```python
from build123d import *

# Parameters (mm, degrees)
SKETCH1_W                                    = 240
SKETCH1_H                                    = 100
BOSS_EXTRUDE1_DEPTH                          = 5
SKETCH2_W                                    = 20
SKETCH2_H                                    = 5
BOSS_EXTRUDE2_DEPTH                          = 5
MIRROR1_AT_THE_SECOND_PLANE_COPY_1_SKETC_W   = 20
MIRROR1_AT_THE_SECOND_PLANE_COPY_1_SKETC_H   = 5
MIRROR1_AT_THE_SECOND_PLANE_COPY_1_DEPTH     = 5
SKETCH3_R                                    = 6
SKETCH3_R_2                                  = 2
BOSS_EXTRUDE3_DEPTH                          = 5
SKETCH4_R                                    = 2.5
CUT_EXTRUDE2_DEPTH                           = 5
MIRROR2_AT_THE_SECOND_PLANE_COPY_1_SKETC_R   = 6
MIRROR2_AT_THE_SECOND_PLANE_COPY_1_SKETC_R_2 = 2
MIRROR2_AT_THE_SECOND_PLANE_COPY_1_DEPTH     = 5
MIRROR2_AT_THE_SECOND_PLANE_COPY_2_SKETC_R   = 2.5
MIRROR2_AT_THE_SECOND_PLANE_COPY_2_DEPTH     = 5


with BuildPart() as part:
    # Sketch1 → Boss-Extrude1 (new body)
    with BuildSketch(Plane.XY):
        Rectangle(SKETCH1_W, SKETCH1_H)
    extrude(amount=BOSS_EXTRUDE1_DEPTH)

    # Sketch2 → Boss-Extrude2 (add)
    with BuildSketch(Plane(origin=(0, 50, 0), x_dir=(1, 0, 0), z_dir=(0, 1, 0))):
        with Locations((50, -2.5)):
            Rectangle(SKETCH2_W, SKETCH2_H)
    boss_extrude2 = extrude(amount=BOSS_EXTRUDE2_DEPTH)

    # Mirror1: Boss-Extrude2 across plane
    add(boss_extrude2.mirror(Plane(origin=(0, 0, 0), x_dir=(0, 0, 1), z_dir=(1, 0, 0))))

    # Mirror1 at the second plane: Boss-Extrude2 across plane
    add(boss_extrude2.mirror(Plane.ZX))

    # Mirror1 at the second plane copy 1 sketc → Mirror1 at the second plane copy 1 (add)
    with BuildSketch(Plane(origin=(0, -50, 0), x_dir=(-1, 0, 0), z_dir=(0, -1, 0))):
        with Locations((50, -2.5)):
            Rectangle(MIRROR1_AT_THE_SECOND_PLANE_COPY_1_SKETC_W, MIRROR1_AT_THE_SECOND_PLANE_COPY_1_SKETC_H)
    extrude(amount=MIRROR1_AT_THE_SECOND_PLANE_COPY_1_DEPTH)

    # Sketch3 → Boss-Extrude3 (add)
    with BuildSketch(Plane.XY.offset(5)):
        with Locations((50, 52.5)):
            Circle(SKETCH3_R)
        with Locations((50, 52.5)):
            Circle(SKETCH3_R_2, mode=Mode.SUBTRACT)
    boss_extrude3 = extrude(amount=-BOSS_EXTRUDE3_DEPTH)

    # Sketch4 → Cut-Extrude2 (cut)
    with BuildSketch(Plane.XY.offset(5)):
        with Locations((50, 52.5)):
            Circle(SKETCH4_R)
    cut_extrude2 = extrude(amount=-CUT_EXTRUDE2_DEPTH, mode=Mode.SUBTRACT)

    # Mirror2: Boss-Extrude3, Cut-Extrude2 across plane
    add(boss_extrude3.mirror(Plane.ZX))
    add(cut_extrude2.mirror(Plane.ZX), mode=Mode.SUBTRACT)

    # Mirror2 at the second plane: Boss-Extrude3, Cut-Extrude2 across plane
    add(boss_extrude3.mirror(Plane(origin=(0, 0, 0), x_dir=(0, 0, 1), z_dir=(1, 0, 0))))
    add(cut_extrude2.mirror(Plane(origin=(0, 0, 0), x_dir=(0, 0, 1), z_dir=(1, 0, 0))), mode=Mode.SUBTRACT)

    # Mirror2 at the second plane copy 1 sketc → Mirror2 at the second plane copy 1 (add)
    with BuildSketch(Plane(origin=(0, 0, 5), x_dir=(-1, 0, 0), z_dir=(0, 0, 1))):
        with Locations((50, 52.5)):
            Circle(MIRROR2_AT_THE_SECOND_PLANE_COPY_1_SKETC_R)
        with Locations((50, 52.5)):
            Circle(MIRROR2_AT_THE_SECOND_PLANE_COPY_1_SKETC_R_2, mode=Mode.SUBTRACT)
    extrude(amount=-MIRROR2_AT_THE_SECOND_PLANE_COPY_1_DEPTH)

    # Mirror2 at the second plane copy 2 sketc → Mirror2 at the second plane copy 2 (cut)
    with BuildSketch(Plane(origin=(0, 0, 5), x_dir=(-1, 0, 0), z_dir=(0, 0, 1))):
        with Locations((50, 52.5)):
            Circle(MIRROR2_AT_THE_SECOND_PLANE_COPY_2_SKETC_R)
    extrude(amount=-MIRROR2_AT_THE_SECOND_PLANE_COPY_2_DEPTH, mode=Mode.SUBTRACT)


solid = part.part
```
Read the model definition and answer for the solid it produces. Units are mm, in the model's axes. A direction names the side the tool comes from. Give positions to 0.01 mm unless a question says otherwise; leave off trailing zeros. Order: outer loops, then holes, each group sorted by start corner. A loop starts at its lowest first (then second) coordinate and runs counter-clockwise, first axis right, second up.
(1) Straight lines are drawn through the part: L1, parallel to Y at x = -50, z = 2.8; L2, parallel to X at y = -52.5, z = 2.35; L3, parallel to Y at x = 37.5, z = 3.8. For each, find the intervals that lie inside material, in ascending order.
(2) Find section D-D (x = -79.5). Give the vertices of the cut face in (y, z).
(3) For a pull along X with two mould halves and no side action, classify faces 1 (the cylindrical face through (-50.1, 58.5, 2.5)), 2 (the flat face through (-60, -52, 3)), 3 (the flat face through (-58, 55, 2)) as released by +X, released by -X, zero draft, split by the parting line, or undercut.
(4) Find section A-A (x = -50). Give the vertices of the cut face in (y, z), plus the area to 3 significant figures.
(5) Given pin 1 (3 mm diameter, centred on x = -27, z = 2, fed in from +Y); pin 2 (8 mm diameter, centred on x = -50, y = 52.5, fed in from -Z); pin 3 (1.5 mm diameter, centred on x = 88, z = 1, fed in from -Y); pin 4 (1.4 mm diameter, centred on x = 57.5, z = 1.5, fed in from -Y), each flat-ended and moving along its own axis, determine where each tip first touches the part or whether it passes through.
(6) Find section C-C (z = 3.8). Give the number of separate pieces and of enclosed holes in the cut face, plus the area to 3 significant figures.
(7) For faces 4 (the cylindrical face through (52.31, -51.54, 2.54)), 5 (the flat face through (-42, 55, 2)), 6 (the flat face through (-90, -50, 2)), 7 (the flat face through (-1, -50, 2)), 8 (the flat face through (90, -50, 2)), determine the directions among +Z, -Z, +X, -X, +Y, -Y from which every point of the face is accessible in a straight line to the end or side of a thin tool.
(8) Find section B-B (y = 52.5). Give the vertices of the cut face in (x, z), plus the area to 3 significant figures.
Result sheet:
1. L1: y = -58.5 to -55, -50 to 50, 55 to 58.5
1. L2: x = -60 to -52.5, -47.5 to -40, 40 to 47.5, 52.5 to 60
1. L3: y = -50 to 50
2. outline: (-50, 0) - (50, 0) - (50, 5) - (-50, 5) - close
3. face 1: undercut
3. face 2: released by -X
3. face 3: zero draft
4. outline: (-58.5, 0) - (-55, 0) - (-55, 5) - (-58.5, 5) - close; (-50, 0) - (50, 0) - (50, 5) - (-50, 5) - close; (55, 0) - (58.5, 0) - (58.5, 5) - (55, 5) - close
4. area: 535 mm2
5. pin 1: stops at y = 50
5. pin 2: stops at z = 0
5. pin 3: stops at y = -50
5. pin 4: stops at y = -55
6. separate pieces: 1
6. enclosed holes: 4
6. area: 24,400 mm2
7. face 4: +Z, -Z
7. face 5: +Z, -Z, +Y
7. face 6: +Z, -Z, -X, -Y
7. face 7: +Z, -Z, -Y
7. face 8: +Z, -Z, +X, -Y
8. outline: (-60, 0) - (-52.5, 0) - (-52.5, 5) - (-60, 5) - close; (-47.5, 0) - (-40, 0) - (-40, 5) - (-47.5, 5) - close; (40, 0) - (47.5, 0) - (47.5, 5) - (40, 5) - close; (52.5, 0) - (60, 0) - (60, 5) - (52.5, 5) - close
8. area: 150 mm2
